Could you check a few things on this model? Use its own coordinates, in mm. A direction names the side the tool comes from. Round coordinates to 2 decimals unless told otherwise and drop trailing zeros. Loops run counter-clockwise (first coordinate to the right, second up) from the corner with the lowest first, then second, coordinate; pieces in that order, holes last. Notation, with made-up numbers: (13, 22) - (63, 22) arc R32 cw to (63, 53) - close; hole circle Ø7 at (24.5, 40.25). An arc over 180 degrees is marked (long way). Use one line per item in the form item = value.
```python
from build123d import *

# Parameters (mm, degrees)
ESQUISSE1_R        = 1.5
ESQUISSE1_W        = 15
ESQUISSE1_H        = 8
BOSS_EXTRU_1_DEPTH = 5


with BuildPart() as part:
    # Esquisse1 → Boss.-Extru.1 (new body)
    with BuildSketch(Plane(origin=(0, 0, 0), x_dir=(1, 0, 0), z_dir=(0, 1, 0))):
        Polygon((78.452994616, 60), (90, 40), (90, 0), (-90, 0), (-90, 60), (-60, 60), (-60, 43), (0, 43), (0, 60), align=None)
        with Locations(Location((-75, 51.5, 0), (0, 0, 270))):
            Circle(ESQUISSE1_R, mode=Mode.SUBTRACT)
        with Locations(Location((8, 51.5, 0), (0, 0, 270))):
            Circle(ESQUISSE1_R, mode=Mode.SUBTRACT)
        with Locations(Location((70, 51.5, 0), (0, 0, 270))):
            Circle(ESQUISSE1_R, mode=Mode.SUBTRACT)
        with Locations(Location((-4, 27.5, 0), (0, 0, 270))):
            Circle(ESQUISSE1_R, mode=Mode.SUBTRACT)
        with Locations((-30, 24)):
            Rectangle(ESQUISSE1_W, ESQUISSE1_H, mode=Mode.SUBTRACT)
    boss_extru_1 = extrude(amount=BOSS_EXTRU_1_DEPTH)

    # Symétrie1: Boss.-Extru.1 across plane
    add(boss_extru_1.mirror(Plane(origin=(-90, 5, 0), x_dir=(1, 0, 0), z_dir=(0, 0, -1))))


solid = part.part
```
1. We'd pull the mould along X, two halves only. Please class faces 1 (the face through (39, 2, 60)), 2 (the face through (-30, 2, -20)), 3 (the face through (84.146, 2.465, -50.14)): +X half, -X half, draft (parallel to the pull), parting line (faces both ways), or undercut.
Solution:
face_1 = draft
face_2 = undercut
face_3 = +X half
2. Please list where these lines run through material, in increasing order: line 1 along X through (y, z) = (4, 27.5); line 2 along X through (y, z) = (3.35, 51.5); line 3 along X through (y, z) = (2.8, 24.5).
Solution:
line_1 = -90 to -37.5, -22.5 to -5.5, -2.5 to 90
line_2 = -90 to -76.5, -73.5 to -60, 0 to 6.5, 9.5 to 68.5, 71.5 to 83.36
line_3 = -90 to -37.5, -22.5 to 90
3. If we section it at B-B, the plane y = 2.5: Count the separate pieces of the cut face and the enclosed holes in it, plus the area to 3 significant figures.
Solution:
separate_pieces = 1
enclosed_holes = 10
area = 19,000 mm^2
4. If we section it at A-A, the plane z = -24: Write out the boundary of the cut face in (x, y).
Solution:
outline = (-90, 0) - (-37.5, 0) - (-37.5, 5) - (-90, 5) - close; (-22.5, 0) - (90, 0) - (90, 5) - (-22.5, 5) - close
5. On a 3-axis mill with a long thin cutter (end or side, diameter ignored), from which of +Z, -Z, +X, -X, +Y, -Y can I reach the whole of each face in a straight line? I mean faces 4 (the face through (-60, 2, 52)), 5 (the face through (-37.5, 2, 24)), 6 (the face through (0, 2, -51)). Say none if no direction works.
Solution:
face_4 = +Z, +Y, -Y
face_5 = +Y, -Y
face_6 = -Z, +Y, -Y
6. For P1, Ø4, axis at x = 70, z = 51.5, coming from the +Y side; P2, Ø1.5, axis at x = -19.5, y = 1.5, coming from the -Z side; P3, Ø1.5, axis at x = -27.5, y = 3.5, coming from the +Z side, each with a flat end and sliding along its axis, tell me the tip position at first contact or that it passes through.
Solution:
P1 = 5
P2 = -43
P3 = 43
